from build123d import *

# Parameters (mm, degrees)
CROQUIS1_R              = 12.5
SALIENTE_EXTRUIR1_DEPTH = 54
SALIENTE_EXTRUIR2_START = 2.5
CROQUIS2_R              = 15
SALIENTE_EXTRUIR2_DEPTH = 2.5
CROQUIS3_R              = 3.75
CORTAR_EXTRUIR2_DEPTH   = 2.5
CROQUIS5_R              = 1.5
CORTAR_EXTRUIR3_DEPTH   = 2.5
CROQUIS9_R              = 1.5
CORTAR_EXTRUIR5_DEPTH   = 2.5


with BuildPart() as part:
    # Croquis1 → Saliente-Extruir1 (new body)
    with BuildSketch(Plane.XY):
        with BuildLine():
            Line((-5.119897429, -1.25), (-15, -1.25))
            Line((-15, -1.25), (-15, 1.25))
            Line((-15, 1.25), (15, 1.25))
            Line((15, 1.25), (15, -1.25))
            Line((15, -1.25), (5.119897429, -1.25))
            Line((5.119897429, -1.25), (5.119897429, -13.25))
            Line((5.119897429, -13.25), (5.119897429, -16.650828027))
            ThreePointArc((5.119897429, -16.650828027), (0, -45.75), (-5.119897429, -16.650828027))
            Line((-5.119897429, -16.650828027), (-5.119897429, -13.25))
            Line((-5.119897429, -13.25), (-5.119897429, -1.25))
        make_face()
        with Locations((0, -30.75)):
            Circle(CROQUIS1_R, mode=Mode.SUBTRACT)
    extrude(amount=SALIENTE_EXTRUIR1_DEPTH)

    # Croquis2 → Saliente-Extruir2 (add)
    with BuildSketch(Plane(origin=(0, 0, 0), x_dir=(-1, 0, 0), z_dir=(0, 0, -1)).offset(SALIENTE_EXTRUIR2_START)):
        with Locations((0, -30.75)):
            Circle(CROQUIS2_R)
    extrude(amount=-SALIENTE_EXTRUIR2_DEPTH)

    # Croquis3 → Cortar-Extruir2 (cut)
    with BuildSketch(Plane(origin=(0, 0, -2.5), x_dir=(-1, 0, 0), z_dir=(0, 0, -1))):
        with Locations((0, -30.75)):
            Circle(CROQUIS3_R)
    extrude(amount=-CORTAR_EXTRUIR2_DEPTH, mode=Mode.SUBTRACT)

    # Croquis5 → Cortar-Extruir3 (cut)
    with BuildSketch(Plane(origin=(0, 0, -2.5), x_dir=(-1, 0, 0), z_dir=(0, 0, -1))):
        with Locations((0, -22.25)):
            Circle(CROQUIS5_R)
        with Locations((0, -39.25)):
            Circle(CROQUIS5_R)
    extrude(amount=-CORTAR_EXTRUIR3_DEPTH, mode=Mode.SUBTRACT)

    # Croquis9 → Cortar-Extruir5 (cut)
    with BuildSketch(Plane(origin=(0, 1.25, 0), x_dir=(1, 0, 0), z_dir=(0, 1, 0))):
        with Locations(Location((-11.25, -50.625, 0), (0, 0, 180))):
            Circle(CROQUIS9_R)
        with Locations((-11.25, -3.375)):
            Circle(CROQUIS9_R)
        with Locations((11.25, -50.625)):
            Circle(CROQUIS9_R)
        with Locations(Location((11.25, -3.375, 0), (0, 0, 180))):
            Circle(CROQUIS9_R)
    extrude(amount=-CORTAR_EXTRUIR5_DEPTH, mode=Mode.SUBTRACT)


solid = part.part
Check sheet for the modelled part. Datum: model origin and axes. Units: mm. A direction names the side the tool comes from. Give positions to 0.01 mm unless a question says otherwise; leave off trailing zeros. Loops run counter-clockwise (first coordinate to the right, second up) from the corner with the lowest first, then second, coordinate; pieces in that order, holes last. Notation, with made-up numbers: M -21,-22 L 31,-22 A12 ccw 31,-13 Z; hole C 32,73.25 d6. An arc over 180 degrees is marked long. Return JSON: item names as keys, results as strings. Group by question number.
1. Tool access check on faces 4 (the cylindrical face through (11.923, -26.995, 26.622)), 5 (the flat face through (5.12, -9, 27)), 6 (the cylindrical face through (0.195, -20.763, -1.268)), 7 (the flat face through (-5.12, -9, 27)), 8 (the cylindrical face through (12.75, 0.02, 3.44)). Record the directions out of +Z, -Z, +X, -X, +Y, -Y that give a thin tool (end or side, any length) a straight path to the whole face; none if there is none.
2. Go/stop test with flat-tipped pins: pin 1 (7.5 mm diameter, centred on x = 3, y = -29, fed in from +Z); pin 2 (5 mm diameter, centred on x = 12, z = 40, fed in from -Y); pin 3 (1.8 mm diameter, centred on x = -11.25, z = 50.625, fed in from +Y). Record where each tip stops, or that it passes through.
3. Mould release check, pull along Z, two halves, no side actions. Record for faces 1 (the flat face through (10, -1.25, 27)), 2 (the cylindrical face through (-12.356, 0.018, 2.361)), 3 (the flat face through (-3, -34, -2.5)): released by +Z, released by -Z, zero draft, split by the parting line, or undercut.
4. Cross-section at A-A on z = 26.5. Record the boundary of the cut face in (x, y), plus the area to 3 significant figures.
5. Cross-section at C-C on y = -30.75. Record the boundary of the cut face in (x, z).
6. Thickness scan on L1, parallel to Y at x = 0, z = -1.45; L2, parallel to Y at x = -7.5, z = 42; L3, parallel to Y at x = -6, z = 22.5. Record the ranges inside material, lowest first.
7. Cross-section at B-B on x = 0. Record the boundary of the cut face in (y, z), plus the area to 3 significant figures.
8. Cross-section at D-D on x = 9. Record the boundary of the cut face in (y, z), plus the area to 3 significant figures.
Return value:
{
 "1": {"face 4": "+Z", "face 5": "+Z, -Z, +X", "face 6": "+Z, -Z", "face 7": "+Z, -Z, -X", "face 8": "+Y"},
 "2": {"pin 1": "z = 0", "pin 2": "y = -42.36", "pin 3": "y = -19.89"},
 "3": {"face 1": "zero draft", "face 2": "undercut", "face 3": "released by -Z"},
 "4": {"outline": "M -15,-1.25 L -5.12,-1.25 L -5.12,-16.65 A15 ccw long 5.12,-16.65 L 5.12,-1.25 L 15,-1.25 L 15,1.25 L -15,1.25 Z; hole C 0,-30.75 d25", "area": "442 mm^2"},
 "5": {"outline": "M -15,-2.5 L -3.75,-2.5 L -3.75,0 L -12.5,0 L -12.5,54 L -15,54 Z; M 3.75,-2.5 L 15,-2.5 L 15,54 L 12.5,54 L 12.5,0 L 3.75,0 Z"},
 "6": {"L1": "-45.75 to -40.75, -37.75 to -34.5, -27 to -23.75, -20.75 to -15.75", "L2": "-43.74 to -40.75, -20.75 to -17.76, -1.25 to 1.25", "L3": "-44.5 to -41.72, -19.78 to -17, -1.25 to 1.25"},
 "7": {"outline": "M -45.75,-2.5 L -40.75,-2.5 L -40.75,0 L -43.25,0 L -43.25,54 L -45.75,54 Z; M -37.75,-2.5 L -34.5,-2.5 L -34.5,0 L -37.75,0 Z; M -27,-2.5 L -23.75,-2.5 L -23.75,0 L -27,0 Z; M -20.75,-2.5 L -15.75,-2.5 L -15.75,0 L 1.25,0 L 1.25,54 L -18.25,54 L -18.25,0 L -20.75,0 Z", "area": "1,230 mm^2"},
 "8": {"outline": "M -42.75,-2.5 L -18.75,-2.5 L -18.75,54 L -22.08,54 L -22.08,0 L -39.42,0 L -39.42,54 L -42.75,54 Z; M -1.25,0 L 1.25,0 L 1.25,54 L -1.25,54 Z", "area": "554 mm^2"}
}
